Here's how the part is built. I have some questions about the finished solid (model axes, mm). A direction names the side the tool comes from. Give positions to 0.01 mm unless a question says otherwise; leave off trailing zeros. Order: outer loops, then holes, each group sorted by start corner. A loop starts at its lowest first (then second) coordinate and runs counter-clockwise, first axis right, second up.
from build123d import *

# Parameters (mm, degrees)
BOSS_EXTRUDE1_DEPTH = 2
SKETCH2_R           = 2.261
CUT_EXTRUDE1_DEPTH  = 4
SKETCH2_3_R         = 2.261
CUT_EXTRUDE2_DEPTH  = 4


with BuildPart() as part:
    # Sketch1 → Boss-Extrude1 (new body)
    with BuildSketch(Plane(origin=(0, 0, 0), x_dir=(1, 0, 0), z_dir=(0, 1, 0))):
        Polygon((-35.69434129, 0), (-35.69434129, 53.3), (58.90182323, 53.3), (61.40182323, 50.8), (61.40182323, 41.31634957), (63.40565871, 41.31634957), (65.90565871, 38.81634957), (65.90565871, 0), align=None)
    extrude(amount=BOSS_EXTRUDE1_DEPTH)

    # Sketch2 → Cut-Extrude1 (cut)
    with BuildSketch(Plane(origin=(0, 2, 0), x_dir=(1, 0, 0), z_dir=(0, 1, 0))):
        with Locations(Location((-20.39434129, 50.7, 0), (0, 0, 270))):
            Circle(SKETCH2_R)
    extrude(amount=-CUT_EXTRUDE1_DEPTH, mode=Mode.SUBTRACT)

    # Sketch2_3 → Cut-Extrude2 (cut)
    with BuildSketch(Plane(origin=(0, 2, 0), x_dir=(1, 0, 0), z_dir=(0, 1, 0))):
        with Locations(Location((-21.69434129, 2.5, 0), (0, 0, 270))):
            Circle(SKETCH2_3_R)
        with Locations(Location((63.201299911, 2.5, 0), (0, 0, 270))):
            Circle(SKETCH2_3_R)
        with Locations(Location((30.40565871, 7.6, 0), (0, 0, 270))):
            Circle(SKETCH2_3_R)
        with Locations(Location((30.40565871, 35.5, 0), (0, 0, 270))):
            Circle(SKETCH2_3_R)
        with Locations(Location((54.50565871, 50.7, 0), (0, 0, 270))):
            Circle(SKETCH2_3_R)
    extrude(amount=-CUT_EXTRUDE2_DEPTH, mode=Mode.SUBTRACT)


solid = part.part
Q1. If we section it at B-B on y = 1: List the corners of the cut face in (x, z) for me.
Filled sheet:
outline: (-35.69, -53.3) - (58.9, -53.3) - (61.4, -50.8) - (61.4, -41.32) - (63.41, -41.32) - (65.91, -38.82) - (65.91, 0) - (-35.69, 0) - close; hole circle Ø4.52 at (-21.69, -2.5); hole circle Ø4.52 at (-20.39, -50.7); hole circle Ø4.52 at (30.41, -35.5); hole circle Ø4.52 at (30.41, -7.6); hole circle Ø4.52 at (54.51, -50.7); hole circle Ø4.52 at (63.2, -2.5)
Q2. If we section it at C-C on z = -45: List the corners of the cut face in (x, y) for me.
Filled sheet:
outline: (-35.69, 0) - (61.4, 0) - (61.4, 2) - (-35.69, 2) - close
Q3. For faces 1 (the face through (61.402, 1, -46)), 2 (the face through (65.443, 1.014, -2.794)), which set-ups out of +Z, -Z, +X, -X, +Y, -Y let a thin tool reach every point of the face, with its end or its side?
Filled sheet:
face 1: -Z, +X, +Y, -Y
face 2: +Y, -Y
Q4. I'm going to push flat-ended pins straight in: P1, Ø1, axis at y = 1.5, z = -46.5, coming from the +X side; P2, Ø5, axis at x = -21.69, z = -2.5, coming from the +Y side. Where does each tip first touch, or does it pass through?
Filled sheet:
P1: stops at x = 61.4
P2: stops at y = 2
Q5. I need wall thicknesses on L1, parallel to X at y = 1.35, z = -50.7; L2, parallel to Z at x = 29.5, y = 0.2; L3, parallel to Z at x = -20, y = 1.8. Which ranges of each line are inside material? Lowest first, please.
Filled sheet:
L1: x = -35.69 to -22.66, -18.13 to 52.24, 56.77 to 61.4
L2: z = -53.3 to -37.57, -33.43 to -9.67, -5.53 to 0
L3: z = -53.3 to -52.93, -48.47 to -4, -1 to 0
Q6. If we section it at A-A on z = -7.6: List the corners of the cut face in (x, y) for me.
Filled sheet:
outline: (-35.69, 0) - (28.14, 0) - (28.14, 2) - (-35.69, 2) - close; (32.67, 0) - (65.91, 0) - (65.91, 2) - (32.67, 2) - close
